Part model, mm, in its own coordinate system. Face numbers are marked on the shaded views. A direction names the side the tool comes from. Round coordinates to 2 decimals unless told otherwise and drop trailing zeros. Loops run counter-clockwise (first coordinate to the right, second up) from the corner with the lowest first, then second, coordinate; pieces in that order, holes last. Notation, with made-up numbers: (24.25, 7.5) - (49.25, 7.5) arc R19 cw to (49.25, 44.5) - close; hole circle Ø6 at (-25.5, 73). An arc over 180 degrees is marked (long way). Write each question's results on one line, items separated by ' | '. Start each with the question number.
(1) Flat gauge pins, fed straight in: P1, Ø6, axis at x = -17.5, y = 11, coming from the +Z side; P2, Ø1, axis at x = -19.5, y = 26.5, coming from the -Z side; P3, Ø3, axis at x = -7.5, z = 5.5, coming from the +Y side; P4, Ø3.5, axis at y = 2, z = 5, coming from the +X side. Where does each tip first touch, or does it go through?
(2) Cut at A-A, the plane z = 12. List the corners of the cut face in (x, y).
(3) Tool access for the marked faces 1 and 2: list every direction of +Z, -Z, +X, -X, +Y, -Y with a clear straight run to the whole face (end or side of a thin tool).
(4) Drill centre lines: L1, parallel to Y at x = -13.75, z = 3; L2, parallel to X at y = 106.5, z = 26; L3, parallel to Y at x = -22, z = 6.5. Where is each one in solid material? Low to high.
(5) Cut at C-C, the plane x = -12. List the corners of the cut face in (y, z), then the cut area to 3 significant figures.
(6) Cut at D-D, the plane z = 27. List the corners of the cut face in (x, y) (3 decimals), then the cut area to 3 significant figures.
(7) Cut at B-B, the plane y = 72.5. List the corners of the cut face in (x, z).
from build123d import *

# Parameters (mm, degrees)
F1_DEPTH = 10
F3_DEPTH = 3
F4_W     = 3
F4_H     = 125
F5_DEPTH = 40
F6_SIZE2 = 24.99999
F6_SIZE  = 39.99999
F7_SIZE  = 25
F9_DEPTH = 25


# Not quite as in the source:
# - a fillet or chamfer is up to 0.001 mm smaller than in the source, because OpenCascade refuses the exact size


with BuildPart() as f1:
    # F0 (on Top) → F1 (new body)
    with BuildSketch(Plane.XY):
        Polygon((0, 3), (0, 0), (10, 0), (20, 20), (20, 145), (17, 145), (17, 20), (10, 3), align=None)
    extrude(amount=F1_DEPTH)

    # F2 (on Front) → F3 (join)
    with BuildSketch(Plane.XZ):
        Polygon((0, 8), (0, 10), (-2, 10), align=None)
    extrude(amount=-F3_DEPTH)

    # F4 (on face) → F5 (join)
    with BuildSketch(Plane.XY.offset(10)):
        with Locations((18.5, 82.5)):
            Rectangle(F4_W, F4_H)
    extrude(amount=F5_DEPTH)

    # F6 (size 40 and 25 in the source; OpenCascade refuses exactly that, so slightly less here)
    f6_edges = [f1.edges().sort_by_distance(p)[0] for p in [
        (18.5, 20, 50),
    ]]
    f6_side = f1.faces().sort_by_distance((18.5, 20, 30))[0]
    chamfer(f6_edges, length=F6_SIZE, length2=F6_SIZE2, reference=f6_side)

    # F7
    f7_edges = [f1.edges().sort_by_distance(p)[0] for p in [
        (18.5, 145, 50),
    ]]
    chamfer(f7_edges, length=F7_SIZE)

    # F8 (on face) → F9 (cut)
    with BuildSketch(Plane.YZ.offset(20)):
        with BuildLine():
            Line((50, 0), (95, 0))
            ThreePointArc((95, 0), (72.5, 35), (50, 0))
        make_face()
    extrude(amount=-F9_DEPTH, mode=Mode.SUBTRACT)


with BuildPart() as f11_1:
    # F11: instance of F1
    add(f1.part.mirror(Plane.YZ.offset(-2)))


solid = f11_1.part
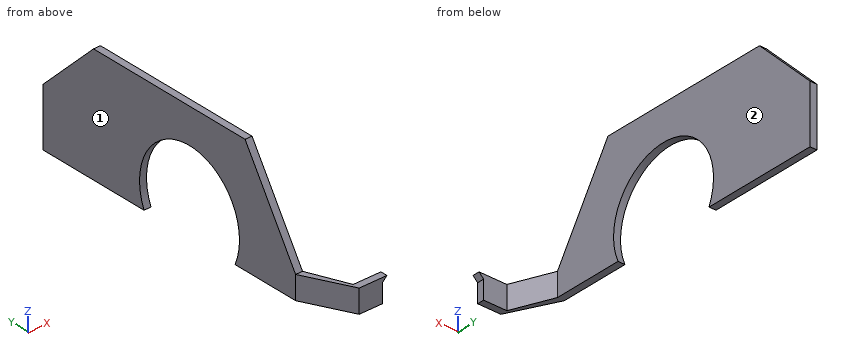
A:
1) P1: z = 10 | P2: through | P3: y = 3 | P4: x = -4
2) outline: (-24, 21.25) - (-21, 21.25) - (-21, 47.83) - (-24, 47.83) - close; (-24, 97.17) - (-21, 97.17) - (-21, 145) - (-24, 145) - close
3) face 1: +Z, -Z, -X, +Y, -Y | face 2: +Z, -Z, +X, +Y
4) L1: 0 to 3 | L2: -24 to -21 | L3: 16 to 48.06, 96.94 to 145
5) outline: (0, 0) - (3, 0) - (3, 10) - (0, 10) - close | area: 30.0 mm2
6) outline: (-24, 30.625) - (-21, 30.625) - (-21, 54.287) - (-24, 54.287) - close; (-24, 90.713) - (-21, 90.713) - (-21, 143) - (-24, 143) - close | area: 228 mm2
7) outline: (-24, 35) - (-21, 35) - (-21, 50) - (-24, 50) - close
